Verification items for this drawing (mm, ordinates from the low corner). A direction names the side the tool comes from. Give positions to 0.01 mm unless a question says otherwise; leave off trailing zeros. Write each loop counter-clockwise with the first axis right and the second up, starting at its lowest first coordinate (ties: lowest second). Pieces come first, ordered by that corner, then holes. Notation, with made-up numbers: (-40, 57.5) -> (-15, 57.5) arc R27 cw to (-15, 83.5) -> close; hole circle Ø4 at (-38.5, -35). An arc over 180 degrees is marked (long way). Use one line per item in the form item = value. Start each with the question number.
(1) Release check for a two-part mould opening along Y. For the marked faces 4, 5 and 6 record: pulls with the +Y half, pulls with the -Y half, needs draft (parallel to the pull), parting line crosses it, or undercut.
(2) Section check A-A, the plane z = 1.5. Record the cut outline in (x, y).
(3) Section check C-C, the plane y = 6.5. Record the cut outline in (x, z), plus the area to 3 significant figures.
(4) Set-up check for the marked faces 1, 2 and 3: record each of +Z, -Z, +X, -X, +Y, -Y from which the full face is reachable in a straight line by a thin tool's end or side.
(5) Scan lines: L1, parallel to Y at x = 31, z = 4.25; L2, parallel to X at y = 11.5, z = 5.5. Record each from-to range of solid material in increasing order.
(6) Depth check by flat-ended pin: pin 1 Ø1 at (y, z) = (5.5, 5) entering from -X; pin 2 Ø2 at (x, z) = (13, 4.5) entering from -Y; pin 3 Ø2 at (y, z) = (10.5, 6.5) entering from +X. Enter the tip coordinate at first touch or a pass-through.
(7) Section check B-B, the plane x = 7. Record the cut outline in (y, z).
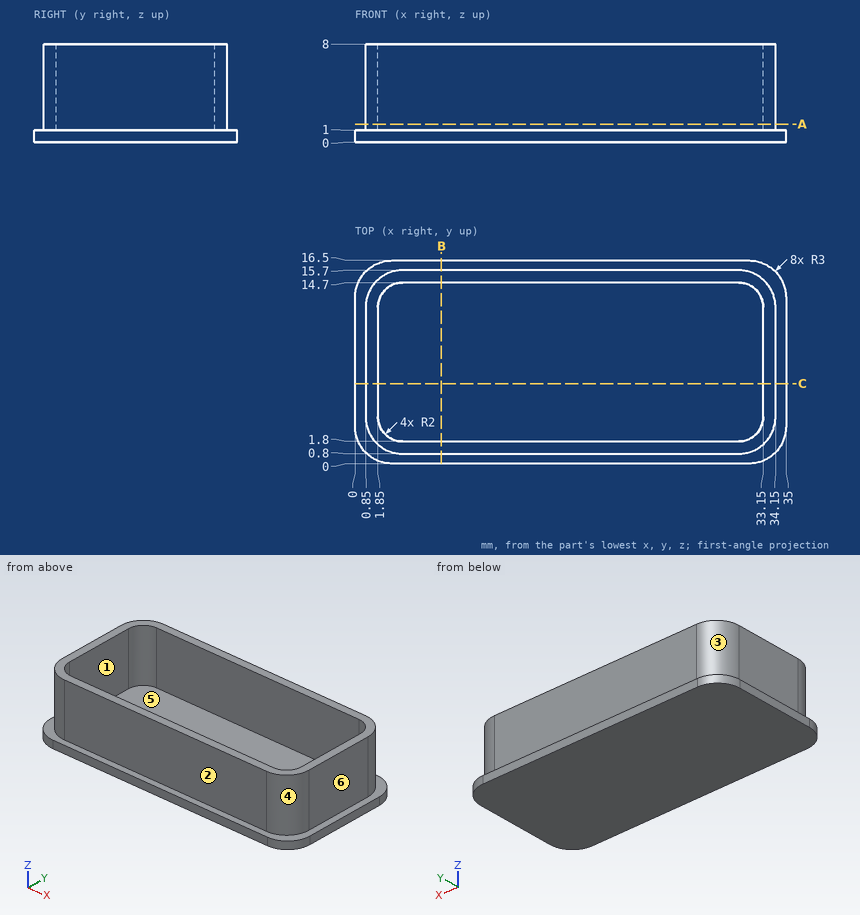
Completed:
q1.face_4 = pulls with the -Y half
q1.face_5 = undercut
q1.face_6 = needs draft
q2.outline = (0.85, 3.8) arc R3 ccw to (3.85, 0.8) -> (31.15, 0.8) arc R3 ccw to (34.15, 3.8) -> (34.15, 12.7) arc R3 ccw to (31.15, 15.7) -> (3.85, 15.7) arc R3 ccw to (0.85, 12.7) -> close; hole (1.85, 3.8) arc R2 ccw to (3.85, 1.8) -> (31.15, 1.8) arc R2 ccw to (33.15, 3.8) -> (33.15, 12.7) arc R2 ccw to (31.15, 14.7) -> (3.85, 14.7) arc R2 ccw to (1.85, 12.7) -> close
q3.outline = (0, 0) -> (35, 0) -> (35, 1) -> (34.15, 1) -> (34.15, 8) -> (33.15, 8) -> (33.15, 1) -> (1.85, 1) -> (1.85, 8) -> (0.85, 8) -> (0.85, 1) -> (0, 1) -> close
q3.area = 49.0 mm²
q4.face_1 = +Z
q4.face_2 = +Z, +X, -X, -Y
q4.face_3 = +Z, -X, +Y
q5.L1 = 0.8 to 1.8, 14.7 to 15.7
q5.L2 = 0.85 to 1.85, 33.15 to 34.15
q6.pin_1 = 0.85
q6.pin_2 = 0.8
q6.pin_3 = 34.15
q7.outline = (0, 0) -> (16.5, 0) -> (16.5, 1) -> (15.7, 1) -> (15.7, 8) -> (14.7, 8) -> (14.7, 1) -> (1.8, 1) -> (1.8, 8) -> (0.8, 8) -> (0.8, 1) -> (0, 1) -> close
